Verification items for the finished model (mm, model axes). Face numbers are marked on the shaded views. Coordinates: 2 decimals unless noted, no trailing zeros. Write each loop counter-clockwise with the first axis right and the second up, starting at its lowest first coordinate (ties: lowest second). Pieces come first, ordered by that corner, then holes. Notation, with made-up numbers: (1, 49) -> (15, 49) arc R9 cw to (15, 58) -> close; hole circle Ø7 at (-11.75, 42). An arc over 180 degrees is marked (long way). Use a Markdown table: item, result. Add a question column.
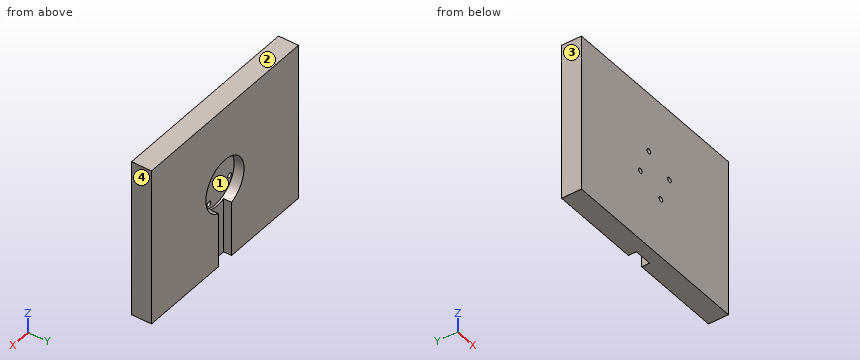
from build123d import *

# Parameters (mm, degrees)
SKETCH1_W                 = 200
SKETCH1_H                 = 160
BASE_DEPTH                = 20
SKETCH2_R                 = 26
LOAD_CELL_CUT_DEPTH       = 10
CUT_WIRE_REACH            = 162
SKETCH6_W                 = 18
SKETCH6_H                 = 8
FILLET6_R                 = 0.1
F_5_0MM_DOWEL_HOLE1_D     = 5
F_5_0MM_DOWEL_HOLE1_DEPTH = 10


with BuildPart() as part:
    # Sketch1 → base (new body)
    with BuildSketch(Plane(origin=(0, 0, 0), x_dir=(1, 0, 0), z_dir=(0, 1, 0))):
        Rectangle(SKETCH1_W, SKETCH1_H)
    extrude(amount=BASE_DEPTH)

    # Sketch2 → load cell cut (cut)
    with BuildSketch(Plane(origin=(0, 20, 0), x_dir=(1, 0, 0), z_dir=(0, 1, 0))):
        Circle(SKETCH2_R)
    extrude(amount=-LOAD_CELL_CUT_DEPTH, mode=Mode.SUBTRACT)

    # Sketch6 → cut wire (cut, up to next)
    with BuildSketch(Plane.XY.offset(-80), mode=Mode.PRIVATE) as cut_wire_sk1:
        with Locations((0, 16)):
            Rectangle(SKETCH6_W, SKETCH6_H)
    cut_wire_tool1 = extrude(cut_wire_sk1.sketch, amount=CUT_WIRE_REACH, mode=Mode.PRIVATE) & part.part
    add(cut_wire_tool1.solids().sort_by_distance((0, 16, -80))[0], mode=Mode.SUBTRACT)

    # Fillet6
    fillet6_edges = [part.edges().sort_by_distance(p)[0] for p in [
        (9, 12, -52.196310918),
        (-9, 12, -52.196310918),
    ]]
    fillet(fillet6_edges, radius=FILLET6_R)

    # Ø5.0mm Dowel Hole1
    with Locations(Plane(origin=(-8.189425453, 0, 19.771021996), x_dir=(0, 0, -1), z_dir=(0, -1, 0))):
        with Locations((0, 0), (11.581596543, 27.960447449), (39.542043992, 16.378850906), (27.960447449, -11.581596543)):
            Hole(F_5_0MM_DOWEL_HOLE1_D / 2, depth=F_5_0MM_DOWEL_HOLE1_DEPTH)


solid = part.part
1) Cross-section at B-B on y = 16. Record the boundary of the cut face in (x, z).
2) Cross-section at C-C on x = 0. Record the boundary of the cut face in (y, z), then the cut area to 3 significant figures.
3) Gauge pin test, flat ends, axial feed: pin 1 (6 mm diameter, centred on x = 19.77, z = 8.19, fed in from +Y); pin 2 (9 mm diameter, centred on x = 2, z = -44, fed in from +Y). Record the tip position at first contact, or that the pin passes through.
4) Release check for a two-part mould opening along X. For the marked faces 1, 2, 3 and 4 record: released by +X, released by -X, zero draft, split by the parting line, or undercut.
5) Thickness scan on L1, parallel to X at y = 13.25, z = -37; L2, parallel to X at y = 7.75, z = -17.5; L3, parallel to Y at x = 1.5, z = 2. Record the ranges inside material, lowest first.
6) Cross-section at A-A on z = -57. Record the boundary of the cut face in (x, y), then the cut area to 3 significant figures.
Returned:
| question | item | result |
|---|---|---|
| 1 | outline | (-100, -80) -> (-9, -80) -> (-9, -24.39) arc R26 cw (long way) to (9, -24.39) -> (9, -80) -> (100, -80) -> (100, 80) -> (-100, 80) -> close |
| 2 | outline | (0, -80) -> (12, -80) -> (12, -26) -> (10, -26) -> (10, 26) -> (20, 26) -> (20, 80) -> (0, 80) -> close |
| 2 | area | 2,250 mm² |
| 3 | pin 1 | stops at y = 10 |
| 3 | pin 2 | stops at y = 12 |
| 4 | face 1 | undercut |
| 4 | face 2 | zero draft |
| 4 | face 3 | released by -X |
| 4 | face 4 | released by +X |
| 5 | L1 | x = -100 to -9, 9 to 100 |
| 5 | L2 | x = -100 to 7.14, 9.23 to 100 |
| 5 | L3 | y = 0 to 10 |
| 6 | outline | (-100, 0) -> (100, 0) -> (100, 20) -> (9, 20) -> (9, 12.1) arc R0.1 cw to (8.9, 12) -> (-8.9, 12) arc R0.1 cw to (-9, 12.1) -> (-9, 20) -> (-100, 20) -> close |
| 6 | area | 3,860 mm² |
